For this review, use the dimensioned drawing (mm, ordinates from the lowest corner) and the shaded views. A direction names the side the tool comes from. Round coordinates to 2 decimals unless told otherwise and drop trailing zeros. Write each loop counter-clockwise with the first axis right and the second up, starting at its lowest first coordinate (ties: lowest second). Pieces come first, ordered by that corner, then holes. Notation, with made-up numbers: M 72,59 L 93,59 A8 ccw 93,69 Z; hole C 75.25,45.25 d5. An arc over 180 degrees is marked long. Answer in a Markdown table with one row per item.
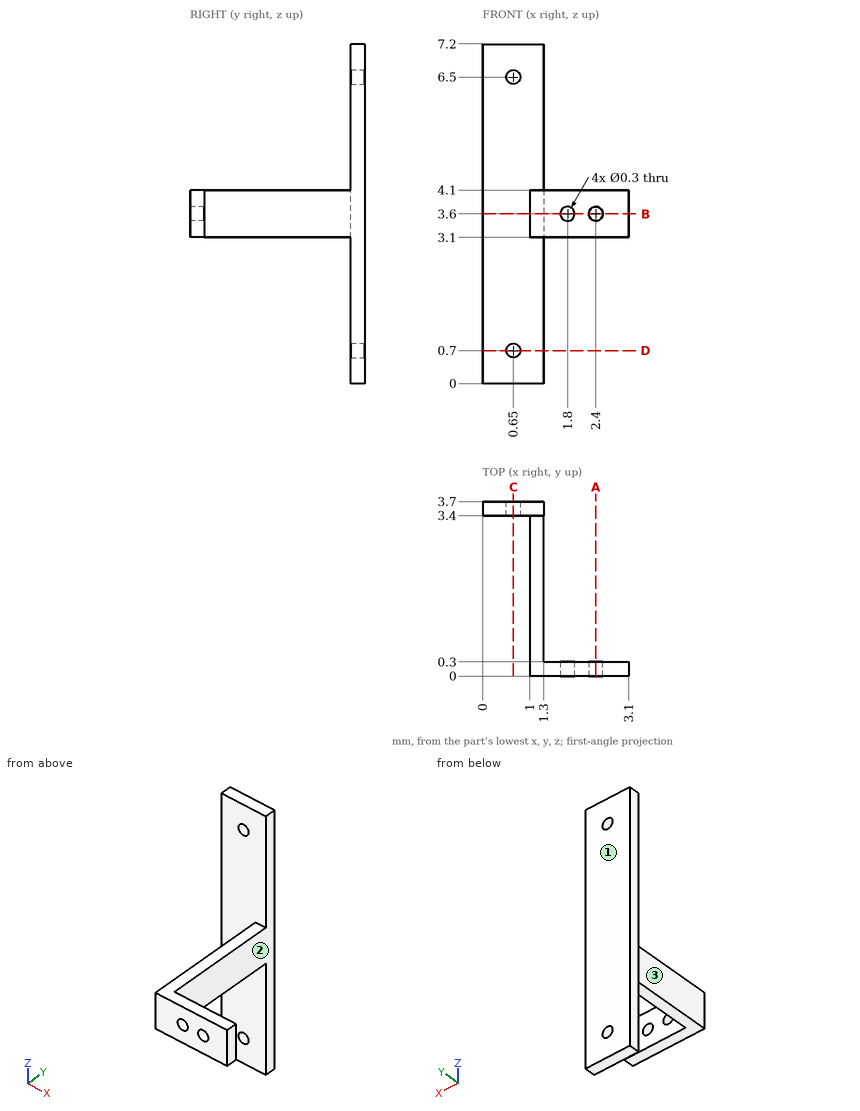
Q1. Take a section at B-B (z = 3.6). State the section outline as (x, y) points, then the cut area to 3 significant figures.
Found:
| item | result |
|---|---|
| outline | M 0,3.4 L 1,3.4 L 1,0 L 1.65,0 L 1.65,0.3 L 1.3,0.3 L 1.3,3.7 L 0,3.7 Z; M 1.95,0 L 2.25,0 L 2.25,0.3 L 1.95,0.3 Z; M 2.55,0 L 3.1,0 L 3.1,0.3 L 2.55,0.3 Z |
| area | 1.77 mm² |
Q2. For probe 1 along Z at (x, y) = (0.65, 3.65); probe 2 along Z at (x, y) = (1.8, 0.25); probe 3 along X at (y, z) = (0.1, 3.6), list the stretches that pass through material, from the lowest coordinate up.
Found:
| item | result |
|---|---|
| probe 1 | 0 to 0.55, 0.85 to 6.35, 6.65 to 7.2 |
| probe 2 | 3.1 to 3.45, 3.75 to 4.1 |
| probe 3 | 1 to 1.65, 1.95 to 2.25, 2.55 to 3.1 |
Q3. Take a section at C-C (x = 0.65). State the section outline as (y, z) points, then the cut area to 3 significant figures.
Found:
| item | result |
|---|---|
| outline | M 3.4,0 L 3.7,0 L 3.7,0.55 L 3.4,0.55 Z; M 3.4,0.85 L 3.7,0.85 L 3.7,6.35 L 3.4,6.35 Z; M 3.4,6.65 L 3.7,6.65 L 3.7,7.2 L 3.4,7.2 Z |
| area | 1.98 mm² |
Q4. Take a section at D-D (z = 0.7). State the section outline as (x, y) points, then the cut area to 3 significant figures.
Found:
| item | result |
|---|---|
| outline | M 0,3.4 L 0.5,3.4 L 0.5,3.7 L 0,3.7 Z; M 0.8,3.4 L 1.3,3.4 L 1.3,3.7 L 0.8,3.7 Z |
| area | 0.300 mm² |
Q5. Machinability: for the marked faces 1, 2 and 3, which of the approach directions +Z, -Z, +X, -X, +Y, -Y give a long, thin tool a straight path to every point of the face, cutting with its end or side? Answer none if there is none.
Found:
| item | result |
|---|---|
| face 1 | +Z, -Z, +X, -X, +Y |
| face 2 | +Z, -Z, +X, +Y |
| face 3 | +Z, -Z, -X, -Y |
Q6. Insertion check: P1, Ø0.5, axis at x = 2, z = 3.5, coming from the +Y side; P2, Ø1.1, axis at y = 1.5, z = 3.5, coming from the -X side; P3, Ø1.7, axis at x = 1.5, y = 1.5, coming from the -Z side. Each pin has a flat end and moves straight along its axis. Give the tip position at first contact, or say it passes through.
Found:
| item | result |
|---|---|
| P1 | y = 0.3 |
| P2 | x = 1 |
| P3 | z = 3.1 |
Q7. Take a section at A-A (x = 2.4). State the section outline as (y, z) points, then the cut area to 3 significant figures.
Found:
| item | result |
|---|---|
| outline | M 0,3.1 L 0.3,3.1 L 0.3,3.45 L 0,3.45 Z; M 0,3.75 L 0.3,3.75 L 0.3,4.1 L 0,4.1 Z |
| area | 0.210 mm² |
